Design review of the part built by this model. Coordinates are the model's own, in mm. A direction names the side the tool comes from. Coordinates: 2 decimals unless noted, no trailing zeros. Loops run counter-clockwise (first coordinate to the right, second up) from the corner with the lowest first, then second, coordinate; pieces in that order, holes last.
from build123d import *

# Parameters (mm, degrees)
ENL_V_MAT_EXTRU_4_DEPTH = 8
ENL_V_MAT_EXTRU_5_DEPTH = 33


with BuildPart() as part:
    # Esquisse4 → Révolution1 (revolve)
    with BuildSketch(Plane.XY):
        Polygon((-10.030612245, 30), (-10.030612245, -10), (-2.030612245, -10), (-2.030612245, -7), (-4.030612245, -7), (-4.030612245, 30), align=None)
    revolve(axis=Axis((-10.030612245, 30, 0), (0, -1, 0)))

    # Esquisse9 → Enlèv. mat.-Extru.4 (cut)
    with BuildSketch(Plane(origin=(0, 30, 0), x_dir=(1, 0, 0), z_dir=(0, 1, 0))):
        Polygon((-12.530612245, 1.5), (-7.530612245, 1.5), (-7.530612245, 0.5), (-7.530612245, -0.5), (-7.530612245, -1.5), (-12.530612245, -1.5), (-12.530612245, -0.5), (-12.530612245, 0.5), align=None)
    extrude(amount=-ENL_V_MAT_EXTRU_4_DEPTH, mode=Mode.SUBTRACT)

    # Esquisse11 → Enlèv. mat.-Extru.5 (cut)
    with BuildSketch(Plane(origin=(0, 30, 0), x_dir=(1, 0, 0), z_dir=(0, 1, 0))):
        Polygon((-10.030612245, 3.75), (-11.530612245, 3.75), (-11.530612245, 6.147265129), (-8.530612245, 6.147265129), (-8.530612245, 3.75), align=None)
        Polygon((-8.530612245, -3.75), (-10.030612245, -3.75), (-11.530612245, -3.75), (-11.530612245, -6.147265129), (-8.530612245, -6.147265129), align=None)
    extrude(amount=-ENL_V_MAT_EXTRU_5_DEPTH, mode=Mode.SUBTRACT)


solid = part.part
Q1. Take a section at C-C, the plane x = -5.25. Write out the cut boundary in (y, z), then the cut area to 3 significant figures.
Q2. Take a section at A-A, the plane z = 0. Write out the cut boundary in (x, y).
Q3. Take a section at B-B, the plane y = 21. Write out the cut boundary in (x, z).
Q4. Machinability: for faces 1 (the flat face through (-10, 30, -3)), 2 (the flat face through (-11.531, 14, 5)), 3 (the flat face through (-10, 26, 1.5)), 4 (the flat face through (-8.531, 14, -5)), which of the approach directions +Z, -Z, +X, -X, +Y, -Y give a long, thin tool a straight path to every point of the face, cutting with its end or side? Answer none if there is none.
Q5. For line 1 (Z direction, x = -9.75, y = 8); line 2 (Y direction, x = -12.75, z = -6); line 3 (X direction, y = 28, z = -0.25), list the stretches that pass through material, from the lowest coordinate up.
Q6. Clearance check with flat-ended pins moving along their axes: pin 1 Ø4 at (x, y) = (-12.5, 16) entering from +Z; pin 2 Ø1 at (x, y) = (-16, 25.5) entering from +Z; pin 3 Ø2.5 at (y, z) = (19, 4.5) entering from +X. State where each tip first meets the part, or that it passes through.
Q7. Take a section at D-D, the plane z = -4.75. Write out the cut boundary in (x, y).
Q8. The part is to be moulded in two halves that separate along Z. For faces 5 (the flat face through (-12.531, 26, 0)), 6 (the flat face through (-10, -3, -5)), 7 (the flat face through (-10, 14, -3.75)), 8 (the cylindrical face through (-16.38, -8.48, -4.87)), say which applies: pulls with the +Z half, pulls with the -Z half, needs draft (parallel to the pull), parting line crosses it, or undercut.
Entries:
1. outline: (-10, -6.41) - (-7, -6.41) - (-7, -3.63) - (30, -3.63) - (30, 3.63) - (-7, 3.63) - (-7, 6.41) - (-10, 6.41) - close
1. area: 307 mm2
2. outline: (-18.03, -10) - (-2.03, -10) - (-2.03, -7) - (-4.03, -7) - (-4.03, 30) - (-7.53, 30) - (-7.53, 22) - (-12.53, 22) - (-12.53, 30) - (-16.03, 30) - (-16.03, -7) - (-18.03, -7) - close
3. outline: (-11.53, -5.81) - (-11.53, -3.75) - (-8.53, -3.75) - (-8.53, -5.81) arc R6 ccw to (-8.53, 5.81) - (-8.53, 3.75) - (-11.53, 3.75) - (-11.53, 5.81) arc R6 ccw to start
4. face 1: +Z, -Z, +X, -X, +Y
4. face 2: +Z, +Y
4. face 3: +Y
4. face 4: -Z, +Y
5. line 1: z = -3.75 to 3.75
5. line 2: y = -10 to -7
5. line 3: x = -16.03 to -12.53, -7.53 to -4.04
6. pin 1: stops at z = 5.81
6. pin 2: stops at z = 2.47
6. pin 3: stops at x = -4.99
7. outline: (-16.47, -10) - (-3.59, -10) - (-3.59, -7) - (-6.36, -7) - (-6.36, 30) - (-8.53, 30) - (-8.53, -3) - (-11.53, -3) - (-11.53, 30) - (-13.7, 30) - (-13.7, -7) - (-16.47, -7) - close
8. face 5: undercut
8. face 6: needs draft
8. face 7: pulls with the -Z half
8. face 8: parting line crosses it
